Read the model definition and answer for the solid it produces. Units are mm, in the model's axes. A direction names the side the tool comes from. Coordinates: 2 decimals unless noted, no trailing zeros. Loops run counter-clockwise (first coordinate to the right, second up) from the corner with the lowest first, then second, coordinate; pieces in that order, holes last. Notation, with made-up numbers: M 54,63 L 67,63 A29 cw 67,93 Z; hole C 58,84 d4. An arc over 180 degrees is marked long. One line per item, written item: value. Start each with the question number.
1. Flat-ended cylindrical pins translate along their axes: pin 1 (0.9 mm diameter, centred on y = 43, z = 1, fed in from +X); pin 2 (2.5 mm diameter, centred on y = -40, z = 1.5, fed in from -X); pin 3 (1.5 mm diameter, centred on x = -32.5, y = -5.5, fed in from -Z). Find the tip coordinate at first contact, or state that the pin passes through.
2. The part is cut by section B-B (z = -8.25). Write down the section's boundary in (x, y).
3. Determine the mould class of faces 1 (the face through (49.527, 41.859, 1.479)), 2 (the face through (10.5, 41, -5)), 3 (the face through (-7.5, 41, -5)) for opening direction X: +X half, -X half, draft (parallel to the pull), parting line (faces both ways), or undercut.
4. The part is cut by section C-C (x = 36). Write down the section's boundary in (y, z).
5. For faces 4 (the face through (6.5, 41, -5)), 5 (the face through (-5, 37, -7)), determine the directions among +Z, -Z, +X, -X, +Y, -Y from which every point of the face is accessible in a straight line to the end or side of a thin tool.
6. Consider probe 1 along X at (y, z) = (30.5, -1.25); probe 2 along Z at (x, y) = (-93.5, 13.5); probe 3 along X at (y, z) = (-34.5, 1). Determine where each line is inside the solid, lowest interval first.
7. The part is cut by section D-D (x = -115). Write down the section's boundary in (y, z).
8. The part is cut by section A-A (x = 87.5). Write down the section's boundary in (y, z), then the cut area to 3 significant figures.
```python
from build123d import *

# Parameters (mm, degrees)
SKETCH_1_W          = 291
SKETCH_1_H          = 105
EXTRUDE_1_DEPTH     = 3
SKETCH_2_W          = 3
SKETCH_2_H          = 26.25
SKETCH_2_W_2        = 48.5
SKETCH_2_H_2        = 3
CUT_EXTRUDE_1_DEPTH = 3
SKETCH_3_R          = 40
SKETCH_3_R_2        = 2.75
CUT_EXTRUDE_2_DEPTH = 3
SKETCH_4_W          = 4
SKETCH_4_H          = 28
EXTRUDE_2_DEPTH     = 14
CUT_EXTRUDE_3_REACH = 167.192


with BuildPart() as part:
    # Эскиз1 → Бобышка-Вытянуть1 (new body)
    with BuildSketch(Plane.XY):
        Rectangle(SKETCH_1_W, SKETCH_1_H)
    extrude(amount=EXTRUDE_1_DEPTH)

    # Эскиз2 → Вырез-Вытянуть1 (cut)
    with BuildSketch(Plane.XY.offset(3)):
        with Locations((-144, -39.375)):
            Rectangle(SKETCH_2_W, SKETCH_2_H)
        with Locations((-144, 13.125)):
            Rectangle(SKETCH_2_W, SKETCH_2_H)
        with Locations((-72.75, -51)):
            Rectangle(SKETCH_2_W_2, SKETCH_2_H_2)
        with Locations((24.25, -51)):
            Rectangle(SKETCH_2_W_2, SKETCH_2_H_2)
        with Locations((121.25, -51)):
            Rectangle(SKETCH_2_W_2, SKETCH_2_H_2)
        with Locations((144, 39.375)):
            Rectangle(SKETCH_2_W, SKETCH_2_H)
        with Locations((144, -13.125)):
            Rectangle(SKETCH_2_W, SKETCH_2_H)
    extrude(amount=-CUT_EXTRUDE_1_DEPTH, mode=Mode.SUBTRACT)

    # Эскиз3 → Вырез-Вытянуть2 (cut)
    with BuildSketch(Plane(origin=(0, 0, 0), x_dir=(-1, 0, 0), z_dir=(0, 0, -1))):
        with Locations((-87.5, 0)):
            Circle(SKETCH_3_R)
        with Locations((-127.5, 40)):
            Circle(SKETCH_3_R_2)
        with Locations((-47.5, 40)):
            Circle(SKETCH_3_R_2)
        with Locations((-47.5, -40)):
            Circle(SKETCH_3_R_2)
        with Locations((-127.5, -40)):
            Circle(SKETCH_3_R_2)
    extrude(amount=-CUT_EXTRUDE_2_DEPTH, mode=Mode.SUBTRACT)

    # Эскиз4 → Бобышка-Вытянуть2 (add)
    with BuildSketch(Plane(origin=(0, 0, 0), x_dir=(-1, 0, 0), z_dir=(0, 0, -1))):
        with Locations((5.5, 38.5)):
            Rectangle(SKETCH_4_W, SKETCH_4_H)
        with Locations((-8.5, 38.5)):
            Rectangle(SKETCH_4_W, SKETCH_4_H)
    extrude(amount=EXTRUDE_2_DEPTH)

    # Вырез-Вытянуть3: up to this face of the body (flat: up to its plane)
    cut_extrude_3_end = Plane(part.part.faces().sort_by_distance((-7.5, 38.5, -7))[0])
    # Эскиз5 → Вырез-Вытянуть3 (cut, up to the picked face)
    with BuildSketch(Plane(origin=(10.5, 0, 0), x_dir=(0, 0, -1), z_dir=(1, 0, 0)), mode=Mode.PRIVATE) as cut_extrude_3_sk1:
        Polygon((0, 24.5), (14, 24.5), (14, 49.5), align=None)
    cut_extrude_3_tool1 = split(extrude(cut_extrude_3_sk1.sketch, amount=-CUT_EXTRUDE_3_REACH, mode=Mode.PRIVATE), bisect_by=cut_extrude_3_end, keep=Keep.BOTH, mode=Mode.PRIVATE)
    add(cut_extrude_3_tool1.solids().sort_by(Axis((10.5, 32.833333, -9.333333), (-1, 0, 0)))[0], mode=Mode.SUBTRACT)


solid = part.part
```
Answer block:
1. pin 1: stops at x = 142.5
1. pin 2: stops at x = -142.5
1. pin 3: stops at z = 0
2. outline: M -7.5,39.23 L -3.5,39.23 L -3.5,52.5 L -7.5,52.5 Z; M 6.5,39.23 L 10.5,39.23 L 10.5,52.5 L 6.5,52.5 Z
3. face 1: undercut
3. face 2: +X half
3. face 3: -X half
4. outline: M -49.5,0 L 52.5,0 L 52.5,3 L -49.5,3 Z
5. face 4: -Z, +Y, -Y
5. face 5: -Z, +X, -X, -Y
6. probe 1: x = -7.5 to -3.5, 6.5 to 10.5
6. probe 2: z = 0 to 3
6. probe 3: x = -142.5 to 67.26, 107.74 to 145.5
7. outline: M -52.5,0 L 52.5,0 L 52.5,3 L -52.5,3 Z
8. outline: M -52.5,0 L -40,0 L -40,3 L -52.5,3 Z; M 40,0 L 52.5,0 L 52.5,3 L 40,3 Z
8. area: 75.0 mm2
